from build123d import *

# Parameters (mm, degrees)
EXTRUDE_1_DEPTH     = 3
SKETCH_2_W          = 13.000000000000007
SKETCH_2_H          = 2.000000000000014
SKETCH_2_W_2        = 12.999999999999993
EXTRUDE_2_DEPTH     = 4
CUT_EXTRUDE_1_REACH = 156.172
SKETCH_3_W          = 10.000000000000021
SKETCH_3_H          = 1.5
SKETCH_3_W_2        = 10
FILLET_1_R          = 1
CHAMFER_1_SIZE      = 4
CHAMFER_2_SIZE      = 3
EXTRUDE_3_DEPTH     = 1
CHAMFER_3_SIZE      = 2
CUT_EXTRUDE_2_REACH = 115.098
CUT_EXTRUDE_3_DEPTH = 1
EXTRUDE_4_DEPTH     = 16.4
CUT_EXTRUDE_4_REACH = 201.064
SKETCH_9_W          = 8.500000000000004
SKETCH_9_H          = 1.5000000000000036
SKETCH_10_W         = 14.5
SKETCH_10_H         = 1.5000000000000284
CUT_EXTRUDE_5_DEPTH = 1
SKETCH_11_W         = 14.496613720637008
SKETCH_11_H         = 3.000000000000007
EXTRUDE_5_DEPTH     = 5
FILLET_2_R          = 2


with BuildPart() as part:
    # 草图1 → 凸台-拉伸1 (new body)
    with BuildSketch(Plane(origin=(0, 0, 0), x_dir=(1, 0, 0), z_dir=(0, 1, 0))):
        Polygon((93.99999999999997, -62.499999999999964), (-94.00000000000001, -62.5), (-94.00000000000003, 62.500000000000014), (93.99999999999997, 62.50000000000004), align=None)
    extrude(amount=-EXTRUDE_1_DEPTH)

    # 草图2 → 凸台-拉伸2 (add)
    with BuildSketch(Plane.XZ.offset(3)):
        with Locations((-67.50000000000003, 58.5)):
            Rectangle(SKETCH_2_W, SKETCH_2_H)
        with Locations((40.49999999999994, 58.5)):
            Rectangle(SKETCH_2_W_2, SKETCH_2_H)
        with Locations((40.49999999999994, -58.5)):
            Rectangle(SKETCH_2_W_2, SKETCH_2_H)
        with Locations((-67.50000000000003, -58.5)):
            Rectangle(SKETCH_2_W, SKETCH_2_H)
    extrude(amount=EXTRUDE_2_DEPTH)

    # 切除-拉伸1: up to this face of the body (flat: up to its plane)
    cut_extrude_1_end = Plane(part.part.faces().sort_by_distance((40.5, -5, -59.5))[0])
    # 草图3 → 切除-拉伸1 (cut, up to the picked face)
    with BuildSketch(Plane.XY.offset(59.500000000000036), mode=Mode.PRIVATE) as cut_extrude_1_sk1:
        with Locations((-67.5, -4.75)):
            Rectangle(SKETCH_3_W, SKETCH_3_H)
    cut_extrude_1_tool1 = split(extrude(cut_extrude_1_sk1.sketch, amount=-CUT_EXTRUDE_1_REACH, mode=Mode.PRIVATE), bisect_by=cut_extrude_1_end, keep=Keep.BOTH, mode=Mode.PRIVATE)
    # 草图3 → 切除-拉伸1 (cut, up to the picked face)
    with BuildSketch(Plane.XY.offset(59.500000000000036), mode=Mode.PRIVATE) as cut_extrude_1_sk2:
        with Locations((40.499999999999986, -4.75)):
            Rectangle(SKETCH_3_W_2, SKETCH_3_H)
    cut_extrude_1_tool2 = split(extrude(cut_extrude_1_sk2.sketch, amount=-CUT_EXTRUDE_1_REACH, mode=Mode.PRIVATE), bisect_by=cut_extrude_1_end, keep=Keep.BOTH, mode=Mode.PRIVATE)
    add(cut_extrude_1_tool1.solids().sort_by(Axis((-67.5, -4.75, 59.5), (0, 0, -1)))[0], mode=Mode.SUBTRACT)
    add(cut_extrude_1_tool2.solids().sort_by(Axis((40.5, -4.75, 59.5), (0, 0, -1)))[0], mode=Mode.SUBTRACT)

    # 圆角1
    fillet_1_edges = [part.edges().sort_by_distance(p)[0] for p in [
        (-74.00000000000003, -7, 58.5),
        (-61.00000000000003, -7, 58.5),
        (33.99999999999995, -7, 58.5),
        (46.99999999999994, -7, 58.5),
        (33.99999999999995, -7, -58.5),
        (46.99999999999994, -7, -58.5),
        (-74.00000000000003, -7, -58.5),
        (-61.00000000000003, -7, -58.5),
    ]]
    fillet(fillet_1_edges, radius=FILLET_1_R)

    # 倒角1
    chamfer_1_edges = [part.edges().sort_by_distance(p)[0] for p in [
        (-94.00000000000003, -1.5, -62.500000000000014),
        (93.99999999999997, -1.5, -62.50000000000004),
        (93.99999999999997, -1.5, 62.499999999999964),
        (-94.00000000000001, -1.5, 62.5),
    ]]
    chamfer(chamfer_1_edges, length=CHAMFER_1_SIZE)

    # 倒角2
    chamfer_2_edges = [part.edges().sort_by_distance(p)[0] for p in [
        (91.99999999999997, 0, -60.50000000000005),
        (-2.842e-14, 0, -62.50000000000003),
        (-92.00000000000004, 0, -60.50000000000002),
        (-94.00000000000001, 0, -7.11e-15),
        (-92.00000000000003, 0, 60.5),
        (-2.842e-14, 0, 62.499999999999986),
        (91.99999999999999, 0, 60.499999999999964),
        (93.99999999999997, 0, -4.974e-14),
    ]]
    chamfer(chamfer_2_edges, length=CHAMFER_2_SIZE - 0.0001)  # a hair under: the kernel refuses the full size

    # 草图4 → 凸台-拉伸3 (add)
    with BuildSketch(Plane.XZ.offset(3)):
        Polygon((-89.99999999999997, -61.00000000000003), (-92.49999999999997, -58.50000000000002), (-92.49999999999999, 58.499999999999964), (-89.99999999999999, 60.999999999999964), (90.00000000000001, 60.99999999999999), (92.50000000000001, 58.49999999999999), (92.50000000000003, -58.5), (90.00000000000003, -61.00000000000001), align=None)
        Polygon((91, -59.49999999999999), (-91, -59.500000000000014), (-91, 59.49999999999998), (91, 59.50000000000001), align=None, mode=Mode.SUBTRACT)
    extrude(amount=EXTRUDE_3_DEPTH)

    # 倒角3
    chamfer_3_edges = [part.edges().sort_by_distance(p)[0] for p in [
        (91, -3.5, -59.49999999999999),
        (-91, -3.5, 59.49999999999998),
        (-91, -3.5, -59.500000000000014),
        (91, -3.5, 59.50000000000001),
    ]]
    chamfer(chamfer_3_edges, length=CHAMFER_3_SIZE)

    # 草图5 → 切除-拉伸2 (cut, up to next)
    with BuildSketch(Plane(origin=(0, 0, 0), x_dir=(1, 0, 0), z_dir=(0, 1, 0)), mode=Mode.PRIVATE) as cut_extrude_2_sk1:
        Polygon((-68.99999999999999, -47.49999999999995), (11.00000000000001, -47.49999999999995), (11.00000000000001, 4.500000000000045), (-68.99999999999999, 4.500000000000047), align=None)
    cut_extrude_2_tool1 = extrude(cut_extrude_2_sk1.sketch, amount=-CUT_EXTRUDE_2_REACH, mode=Mode.PRIVATE) & part.part
    # 草图5 → 切除-拉伸2 (cut, up to next)
    with BuildSketch(Plane(origin=(0, 0, 0), x_dir=(1, 0, 0), z_dir=(0, 1, 0)), mode=Mode.PRIVATE) as cut_extrude_2_sk2:
        Polygon((2.249999999999944, 40.99999999999997), (10.749999999999943, 40.99999999999997), (10.749999999999941, 49.49999999999997), (2.2499999999999423, 49.499999999999964), align=None)
    cut_extrude_2_tool2 = extrude(cut_extrude_2_sk2.sketch, amount=-CUT_EXTRUDE_2_REACH, mode=Mode.PRIVATE) & part.part
    # 草图5 → 切除-拉伸2 (cut, up to next)
    with BuildSketch(Plane(origin=(0, 0, 0), x_dir=(1, 0, 0), z_dir=(0, 1, 0)), mode=Mode.PRIVATE) as cut_extrude_2_sk3:
        with BuildLine():
            Line((61.79999999999998, 62.50000000000004), (81.99999999999997, 62.50000000000004))
            Line((81.99999999999997, 62.50000000000004), (81.99999999999997, 48.50000000000004))
            ThreePointArc((81.99999999999997, 48.50000000000004), (81.41421356237306, 47.08578643762695), (79.99999999999997, 46.50000000000004))
            Line((79.99999999999997, 46.50000000000004), (63.79999999999998, 46.50000000000004))
            ThreePointArc((63.79999999999998, 46.50000000000004), (62.38578643762689, 47.08578643762695), (61.79999999999998, 48.50000000000004))
            Line((61.79999999999998, 48.50000000000004), (61.79999999999998, 62.50000000000004))
        make_face()
    cut_extrude_2_tool3 = extrude(cut_extrude_2_sk3.sketch, amount=-CUT_EXTRUDE_2_REACH, mode=Mode.PRIVATE) & part.part
    # 草图5 → 切除-拉伸2 (cut, up to next)
    with BuildSketch(Plane(origin=(0, 0, 0), x_dir=(1, 0, 0), z_dir=(0, 1, 0)), mode=Mode.PRIVATE) as cut_extrude_2_sk4:
        with BuildLine():
            Line((22.500000000000018, 9.300000000000042), (78.49999999999999, 9.300000000000042))
            ThreePointArc((78.49999999999999, 9.300000000000042), (79.91421356237309, 8.714213562373137), (80.5, 7.300000000000027))
            Line((80.5, 7.300000000000027), (80.50000000000001, -46.199999999999946))
            ThreePointArc((80.50000000000001, -46.199999999999946), (79.9142135623731, -47.61421356237305), (78.5, -48.19999999999996))
            Line((78.5, -48.19999999999996), (22.500000000000025, -48.19999999999996))
            ThreePointArc((22.500000000000025, -48.19999999999996), (21.085786437626915, -47.61421356237305), (20.500000000000007, -46.199999999999946))
            Line((20.500000000000007, -46.199999999999946), (20.5, 7.300000000000027))
            ThreePointArc((20.5, 7.300000000000027), (21.085786437626904, 8.714213562373137), (22.500000000000018, 9.300000000000042))
        make_face()
    cut_extrude_2_tool4 = extrude(cut_extrude_2_sk4.sketch, amount=-CUT_EXTRUDE_2_REACH, mode=Mode.PRIVATE) & part.part
    add(cut_extrude_2_tool1.solids().sort_by_distance((-29, 0, 21.5))[0], mode=Mode.SUBTRACT)
    add(cut_extrude_2_tool2.solids().sort_by_distance((6.5, 0, -45.25))[0], mode=Mode.SUBTRACT)
    add(cut_extrude_2_tool3.solids().sort_by_distance((71.9, 0, -54.540337))[0], mode=Mode.SUBTRACT)
    add(cut_extrude_2_tool4.solids().sort_by_distance((50.5, 0, 19.45))[0], mode=Mode.SUBTRACT)

    # 草图7 → 切除-拉伸3 (cut)
    with BuildSketch(Plane.XZ.offset(4)):
        Polygon((-92.49999999999999, 58.499999999999964), (-89.99999999999994, 58.499999999999964), (-91, 57.49999999999998), (-91, -57.49999999999998), (-89.99999999999996, -58.50000000000002), (-92.49999999999997, -58.50000000000002), align=None)
    extrude(amount=-CUT_EXTRUDE_3_DEPTH, mode=Mode.SUBTRACT)

    # 草图8 → 凸台-拉伸4 (add)
    with BuildSketch(Plane.XZ.offset(3)):
        Polygon((-94.00000000000003, 58.349999999999966), (-91.00000000000003, 58.349999999999966), (-91.00000000000001, -58.35000000000003), (-94.00000000000001, -58.35000000000003), align=None)
    extrude(amount=EXTRUDE_4_DEPTH)

    # 草图9 → 切除-拉伸4 (cut, up to next)
    with BuildSketch(Plane.ZY.offset(94.00000000000003), mode=Mode.PRIVATE) as cut_extrude_4_sk1:
        Polygon((-14.25000000000002, -19.4), (-4.250000000000012, -19.4), (-4.250000000000012, -10.399999999999999), (-14.250000000000012, -10.399999999999999), align=None)
    cut_extrude_4_tool1 = extrude(cut_extrude_4_sk1.sketch, amount=-CUT_EXTRUDE_4_REACH, mode=Mode.PRIVATE) & part.part
    # 草图9 → 切除-拉伸4 (cut, up to next)
    with BuildSketch(Plane.ZY.offset(94.00000000000003), mode=Mode.PRIVATE) as cut_extrude_4_sk2:
        Polygon((52.24999999999998, -19.4), (38.54999999999998, -19.4), (38.54999999999998, -15.399999999999999), (52.24999999999998, -15.399999999999997), align=None)
    cut_extrude_4_tool2 = extrude(cut_extrude_4_sk2.sketch, amount=-CUT_EXTRUDE_4_REACH, mode=Mode.PRIVATE) & part.part
    # 草图9 → 切除-拉伸4 (cut, up to next)
    with BuildSketch(Plane.ZY.offset(94.00000000000003), mode=Mode.PRIVATE) as cut_extrude_4_sk3:
        Polygon((0.19999999999998752, -19.4), (0.19999999999998752, -16.9), (5.199999999999988, -16.9), (5.1999999999999895, -19.4), align=None)
    cut_extrude_4_tool3 = extrude(cut_extrude_4_sk3.sketch, amount=-CUT_EXTRUDE_4_REACH, mode=Mode.PRIVATE) & part.part
    # 草图9 → 切除-拉伸4 (cut, up to next)
    with BuildSketch(Plane.ZY.offset(94.00000000000003), mode=Mode.PRIVATE) as cut_extrude_4_sk4:
        with Locations((32.24999999999998, -18.65)):
            Rectangle(SKETCH_9_W, SKETCH_9_H)
    cut_extrude_4_tool4 = extrude(cut_extrude_4_sk4.sketch, amount=-CUT_EXTRUDE_4_REACH, mode=Mode.PRIVATE) & part.part
    add(cut_extrude_4_tool1.solids().sort_by_distance((-94, -14.9, -9.25))[0], mode=Mode.SUBTRACT)
    add(cut_extrude_4_tool2.solids().sort_by_distance((-94, -17.4, 45.4))[0], mode=Mode.SUBTRACT)
    add(cut_extrude_4_tool3.solids().sort_by_distance((-94, -18.15, 2.7))[0], mode=Mode.SUBTRACT)
    add(cut_extrude_4_tool4.solids().sort_by_distance((-94, -18.65, 32.25))[0], mode=Mode.SUBTRACT)

    # 草图10 → 切除-拉伸5 (cut)
    with BuildSketch(Plane.XZ.offset(4)):
        with Locations((54.54999999999998, -60.25000000000001)):
            Rectangle(SKETCH_10_W, SKETCH_10_H)
    extrude(amount=-CUT_EXTRUDE_5_DEPTH, mode=Mode.SUBTRACT)

    # 草图11 → 凸台-拉伸5 (add)
    with BuildSketch(Plane.XZ.offset(3)):
        with Locations((54.551693139681475, -61.00000000000004)):
            Rectangle(SKETCH_11_W, SKETCH_11_H)
    extrude(amount=EXTRUDE_5_DEPTH)

    # 圆角2
    fillet_2_edges = [part.edges().sort_by_distance(p)[0] for p in [
        (81.99999999999997, 0, -54.000050000000044),
        (81.41421356237306, 0, -47.08578643762695),
        (71.89999999999998, 0, -46.50000000000004),
        (62.38578643762689, 0, -47.08578643762695),
        (81.99999999999997, -1.499950000000006, -61.00005000000004),
        (61.79999999999998, -5.49995, -62.50000000000004),
        (61.79999999999998, -1.4999500000000077, -61.00005000000003),
        (61.79999999999998, 0, -54.000050000000044),
    ]]
    fillet(fillet_2_edges, radius=FILLET_2_R)


solid = part.part
Model file for the job. Use its own axes, mm. A direction names the side the tool comes from. Give positions to 0.01 mm unless a question says otherwise; leave off trailing zeros. Use a Markdown table: item, result. Add a question column.
(1) Tool access for faces 1 (the flat face through (1, 0, -14)), 2 (the flat face through (40, -6, -57.5)), 3 (the cylindrical face through (82.57, -1.9, -60.55)): list every direction of +Z, -Z, +X, -X, +Y, -Y with a clear straight run to the whole face (end or side of a thin tool).
(2) Mould opens along X. For faces 4 (the flat face through (91.1, -1.8, 59.7)), 5 (the flat face through (-91.2, -1.8, -59.6)), 6 (the flat face through (54, -5, -59.5)) say: +X half, -X half, draft (parallel to the pull), parting line (faces both ways), or undercut.
(3) Drop flat-ended pins along their axis: pin 1 Ø1.6 at (y, z) = (-4, -58) entering from +X; pin 2 Ø0.9 at (y, z) = (-5, -61) entering from -X; pin 3 Ø8 at (x, z) = (-39.5, -18.5) entering from +Y; pin 4 Ø2.5 at (y, z) = (-1, 11.5) entering from +X. Give the stop position or say it passes through.
(4) Wall check: line 1 along X through (y, z) = (-2, 18); line 2 along Y through (x, z) = (72.5, -17.5); line 3 along Z through (x, y) = (-45.5, -3.5). Give the ranges that are in metal, low to high.
(5) Slice it at A-A on z = 33.5. Give the number of separate pieces and of enclosed holes in the cut face, and give its area (3 significant figures).
Filled sheet:
| question | item | result |
|---|---|---|
| 1 | face 1 | +Z, -Z, +X, -X, +Y |
| 1 | face 2 | -Y |
| 1 | face 3 | -Z, +Y |
| 2 | face 4 | +X half |
| 2 | face 5 | -X half |
| 2 | face 6 | undercut |
| 3 | pin 1 | x = 92.5 |
| 3 | pin 2 | x = 47.3 |
| 3 | pin 3 | y = 0 |
| 3 | pin 4 | x = 93.25 |
| 4 | line 1 | -93 to -69, 11 to 20.5, 80.5 to 93 |
| 4 | line 2 | -3 to 0 |
| 4 | line 3 | -61 to -59.5, 59.5 to 61 |
| 5 | separate pieces | 3 |
| 5 | enclosed holes | 0 |
| 5 | area | 181 mm2 |
